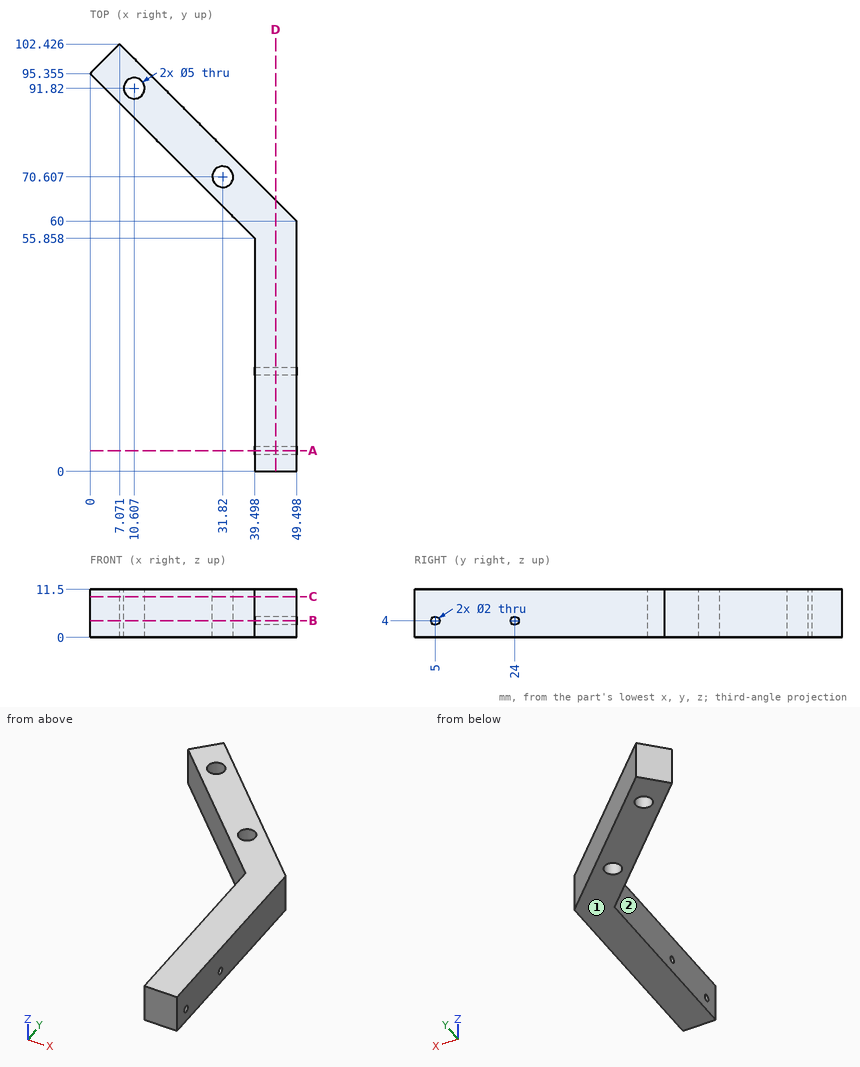
Design review of the part shown in the three views and the two pictorial views. Dimensions are in mm from the part's minimum x, y and z. A direction names the side the tool comes from. Coordinates: 2 decimals unless noted, no trailing zeros. Order: outer loops, then holes, each group sorted by start corner. A loop starts at its lowest first (then second) coordinate and runs counter-clockwise, first axis right, second up.
1) Clearance check with flat-ended pins moving along their axes: pin 1 (1 mm diameter, centred on y = 61.5, z = 6, fed in from -X) (1 decimal); pin 2 (3 mm diameter, centred on x = 37, z = 8, fed in from +Y); pin 3 (3.5 mm diameter, centred on y = 38, z = 7, fed in from -X). State where each tip first meets the part, or that it passes through.
2) Take a section at A-A, the plane y = 5. Give the boundary of the cut face in (x, z).
3) For the marked faces 1 and 2, list the 3-axis set-ups (+Z, -Z, +X, -X, +Y, -Y) from which the entire face can be reached by the end or side of a thin tool; tool diameter is ignored.
4) Take a section at C-C, the plane z = 9.75. Give the boundary of the cut face in (x, y) (1 decimal), and give its area (3 significant figures).
5) Take a section at B-B, the plane z = 4. Give the boundary of the cut face in (x, y) (1 decimal), and give its area (3 significant figures).
6) Wall thickness on line 1 along Y through (x, z) = (43.5, 4) (1 decimal); line 2 along X through (y, z) = (70, 6.5) (1 decimal); line 3 along Y through (x, z) = (46.5, 4) (1 decimal): over which ranges is each line inside the solid? List them lowest first.
7) Take a section at D-D, the plane x = 44.5. Give the boundary of the cut face in (y, z).
Returned:
1. pin 1: stops at x = 33.4
1. pin 2: stops at y = 74
1. pin 3: stops at x = 39.5
2. outline: (39.5, 0) - (49.5, 0) - (49.5, 3) - (39.5, 3) - close; (39.5, 5) - (49.5, 5) - (49.5, 11.5) - (39.5, 11.5) - close
3. face 1: -Z, +X, -X, +Y, -Y
3. face 2: +Z, -Z, -X, -Y
4. outline: (0, 95.4) - (39.5, 55.9) - (39.5, 0) - (49.5, 0) - (49.5, 60) - (7.1, 102.4) - close; hole circle Ø5 at (10.6, 91.8); hole circle Ø5 at (31.8, 70.6)
4. area: 1,120 mm2
5. outline: (0, 95.4) - (39.5, 55.9) - (39.5, 25) - (49.5, 25) - (49.5, 60) - (7.1, 102.4) - close; (39.5, 0) - (49.5, 0) - (49.5, 4) - (39.5, 4) - close; (39.5, 6) - (49.5, 6) - (49.5, 23) - (39.5, 23) - close; hole circle Ø5 at (10.6, 91.8); hole circle Ø5 at (31.8, 70.6)
5. area: 1,080 mm2
6. line 1: y = 0 to 4, 6 to 23, 25 to 66
6. line 2: x = 25.4 to 29.4, 34.2 to 39.5
6. line 3: y = 0 to 4, 6 to 23, 25 to 63
7. outline: (0, 0) - (65, 0) - (65, 11.5) - (0, 11.5) - close; hole circle Ø2 at (5, 4); hole circle Ø2 at (24, 4)
